Part model, mm, in its own coordinate system. A direction names the side the tool comes from. Round coordinates to 2 decimals unless told otherwise and drop trailing zeros. Order: outer loops, then holes, each group sorted by start corner. A loop starts at its lowest first (then second) coordinate and runs counter-clockwise, first axis right, second up. Notation, with made-up numbers: M -6,21.5 L 43,21.5 A26 ccw 43,46.5 Z; hole C -17,59 d9. An arc over 180 degrees is marked long. Write each question's results on one line, items separated by ' | '. Start each with the question number.
1. Band-saw the part on D-D, the plane y = 2.5. List the corners of the cut face in (x, z).
2. Two-plate mould, pull along X, no slides. Class faces 1 (the face through (5, 0, 0)), 2 (the face through (40.17, 4.19, 0.09)), 3 (the face through (24, 8.89, 0)), 4 (the face through (50.8, 6, 0)): +X half, -X half, draft (parallel to the pull), parting line (faces both ways), or undercut.
3. Band-saw the part on A-A, the plane z = 1. List the corners of the cut face in (x, y) (3 decimals), then the cut area to 3 significant figures.
4. Band-saw the part on B-B, the plane x = 6.35. List the corners of the cut face in (y, z).
5. Probe L1, parallel to X at y = 3.25, z = -1.25; L2, parallel to X at y = 1, z = -4; L3, parallel to X at y = 5, z = -0.5. List the from-to ranges inside material, lowest first. Write a range as [from, to].
6. Band-saw the part on C-C, the plane y = 6.35. List the corners of the cut face in (x, z), then the cut area to 3 significant figures.
7. Which spindle directions (+Z, -Z, +X, -X, +Y, -Y) get a long thin tool onto all of the face, cutting with end or side? Do faces 5 (the face through (39.497, 9.221, 0.089)), 6 (the face through (13.725, 4.507, 0.089)), 7 (the face through (25.8, 9.3, 6.35)). Say none if no direction does.
8. Drop flat-ended pins along their axis: pin 1 Ø1.5 at (x, z) = (29, 0) entering from -Y; pin 2 Ø1 at (x, y) = (16, 6) entering from +Z. Give the stop position or say it passes through.
```python
from build123d import *

# Parameters (mm, degrees)
SKETCH2_R           = 2.54
BOSS_EXTRUDE1_DEPTH = 6.35


with BuildPart() as part:
    # Sketch2 → Boss-Extrude1 (new, symmetric)
    with BuildSketch(Plane.XY):
        Polygon((0, 0), (0, 12.7), (50.8, 12.7), (50.8, 0), (46.99, 0), (41.124121265, 10.16), (37.824564477, 8.255), (42.590590949, 0), (38.780590949, 0), (29.890590949, 8.89), (17.190590949, 8.89), (10.16, 0), align=None)
        with Locations((6.35, 6.35)):
            Circle(SKETCH2_R, mode=Mode.SUBTRACT)
    extrude(amount=BOSS_EXTRUDE1_DEPTH, both=True)


solid = part.part
```
Solution:
1) outline: M 0,-6.35 L 12.14,-6.35 L 12.14,6.35 L 0,6.35 Z; M 36.28,-6.35 L 41.15,-6.35 L 41.15,6.35 L 36.28,6.35 Z; M 45.55,-6.35 L 50.8,-6.35 L 50.8,6.35 L 45.55,6.35 Z
2) face 1: draft | face 2: undercut | face 3: undercut | face 4: +X half
3) outline: M 0,0 L 10.16,0 L 17.191,8.89 L 29.891,8.89 L 38.781,0 L 42.591,0 L 37.825,8.255 L 41.124,10.16 L 46.99,0 L 50.8,0 L 50.8,12.7 L 0,12.7 Z; hole C 6.35,6.35 d5.08 | area: 401 mm^2
4) outline: M 0,-6.35 L 3.81,-6.35 L 3.81,6.35 L 0,6.35 Z; M 8.89,-6.35 L 12.7,-6.35 L 12.7,6.35 L 8.89,6.35 Z
5) L1: [0, 12.73], [35.53, 40.71], [45.11, 50.8] | L2: [0, 10.95], [37.78, 42.01], [46.41, 50.8] | L3: [0, 4.2], [8.5, 14.11], [33.78, 39.7], [44.1, 50.8]
6) outline: M 0,-6.35 L 3.81,-6.35 L 3.81,6.35 L 0,6.35 Z; M 8.89,-6.35 L 15.18,-6.35 L 15.18,6.35 L 8.89,6.35 Z; M 32.43,-6.35 L 38.92,-6.35 L 38.92,6.35 L 32.43,6.35 Z; M 43.32,-6.35 L 50.8,-6.35 L 50.8,6.35 L 43.32,6.35 Z | area: 306 mm^2
7) face 5: +Z, -Z | face 6: +Z, -Z, -Y | face 7: +Z, +X, -X, +Y, -Y
8) pin 1: y = 8.89 | pin 2: through
